```python
from build123d import *

# Parameters (mm, degrees)
F0_R     = 9
F1_DEPTH = 1
F2_R     = 5.625
F3_DEPTH = 7.4
F4_R     = 9
F5_DEPTH = 1
F7_D     = 4


with BuildPart() as f1:
    # F0 (on Top) → F1 (new body)
    with BuildSketch(Plane.XY):
        Circle(F0_R)
    extrude(amount=F1_DEPTH)

    # F2 (on face) → F3 (join)
    with BuildSketch(Plane.XY.offset(1)):
        Circle(F2_R)
    extrude(amount=F3_DEPTH)

    # F4 (on face) → F5 (join)
    with BuildSketch(Plane.XY.offset(8.4)):
        Circle(F4_R)
    extrude(amount=F5_DEPTH)

    # F7 (through all)
    with Locations(Plane.XY.offset(9.4)):
        with Locations((0, 0)):
            Hole(F7_D / 2)


solid = f1.part
```
Check sheet for the modelled part. Datum: model origin and axes. Units: mm. A direction names the side the tool comes from. Round coordinates to 2 decimals unless told otherwise and drop trailing zeros. Order: outer loops, then holes, each group sorted by start corner. A loop starts at its lowest first (then second) coordinate and runs counter-clockwise, first axis right, second up. Notation, with made-up numbers: (-29.75, 71) -> (-12.75, 71) arc R30 ccw to (-12.75, 94) -> close; hole circle Ø8 at (81, -20). An arc over 180 degrees is marked (long way). One line per item, written item: value. Start each with the question number.
Q1. Cross-section at A-A (x = 0). Record the boundary of the cut face in (y, z) (3 decimals).
Q2. Mould release check, pull along Z, two halves, no side actions. Record for faces 1 (the face through (2, -2, 0)), 2 (the face through (-1.172, 8.923, 0.493)), 3 (the face through (2.6, -4.99, 4.65)): pulls with the +Z half, pulls with the -Z half, needs draft (parallel to the pull), parting line crosses it, or undercut.
Q3. Thickness scan on line 1 (Z direction, x = -8, y = -3.75); line 2 (Y direction, x = 0, z = 7.25) (3 decimals); line 3 (X direction, y = -1.5, z = 6.5). Record the ranges inside material, lowest first.
Q4. Cross-section at C-C (z = 2.5). Record the boundary of the cut face in (x, y) (3 decimals).
Q5. Gauge pin test, flat ends, axial feed: pin 1 Ø2 at (y, z) = (-0.5, 1) entering from +X; pin 2 Ø2 at (x, z) = (6, 3.5) entering from +Y; pin 3 Ø2 at (y, z) = (3, 6) entering from +X; pin 4 Ø1 at (x, z) = (7, 4) entering from +Y (3 decimals). Record the tip position at first contact, or that the pin passes through.
Q6. Cross-section at D-D (x = -3.25). Record the boundary of the cut face in (y, z).
Q7. Set-up check for faces 4 (the face through (0, -6, 1)), 5 (the face through (0, -2, 5)): record each of +Z, -Z, +X, -X, +Y, -Y from which the full face is reachable in a straight line by a thin tool's end or side.
Completed:
1. outline: (-9, 0) -> (-2, 0) -> (-2, 9.4) -> (-9, 9.4) -> (-9, 8.4) -> (-5.625, 8.4) -> (-5.625, 1) -> (-9, 1) -> close; (2, 0) -> (9, 0) -> (9, 1) -> (5.625, 1) -> (5.625, 8.4) -> (9, 8.4) -> (9, 9.4) -> (2, 9.4) -> close
2. face 1: pulls with the -Z half
2. face 2: needs draft
2. face 3: undercut
3. line 1: z = 0 to 1, 8.4 to 9.4
3. line 2: y = -5.625 to -2, 2 to 5.625
3. line 3: x = -5.42 to -1.32, 1.32 to 5.42
4. outline: circle Ø11.25 at (0, 0); hole circle Ø4 at (0, 0)
5. pin 1: stops at x = 9
5. pin 2: stops at y = 2.58
5. pin 3: stops at x = 5.26
5. pin 4: passes through
6. outline: (-8.39, 0) -> (8.39, 0) -> (8.39, 1) -> (4.59, 1) -> (4.59, 8.4) -> (8.39, 8.4) -> (8.39, 9.4) -> (-8.39, 9.4) -> (-8.39, 8.4) -> (-4.59, 8.4) -> (-4.59, 1) -> (-8.39, 1) -> close
7. face 4: none
7. face 5: +Z, -Z
